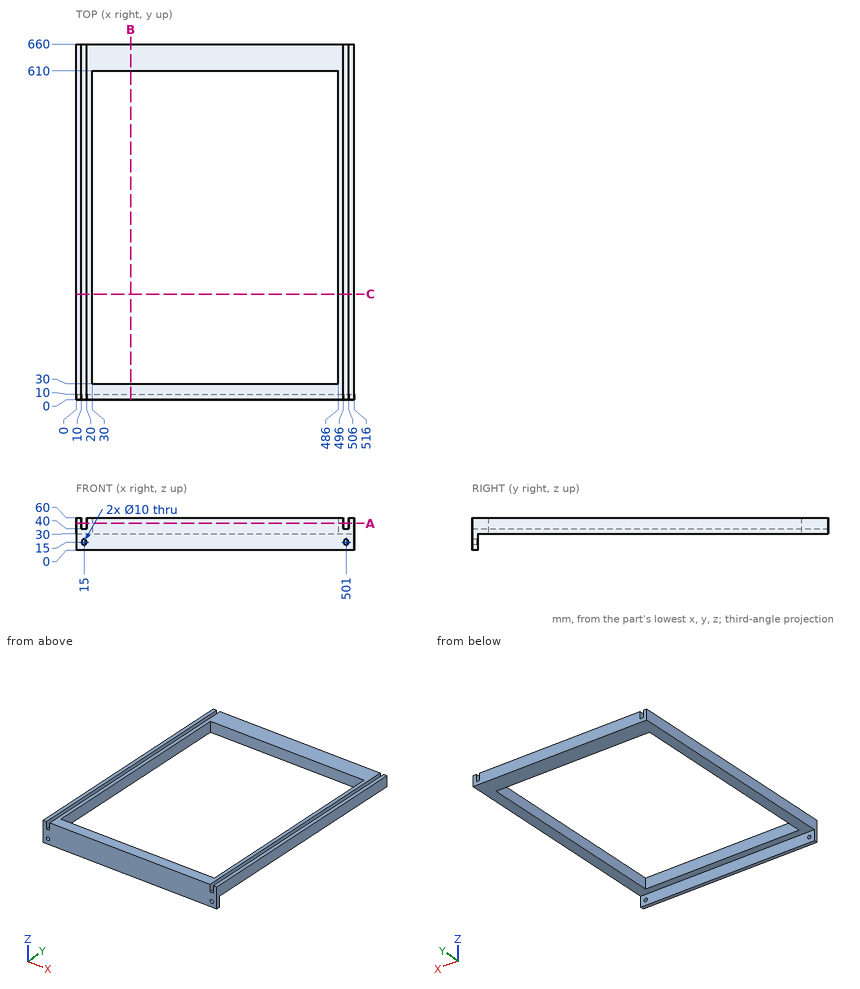
The figure shows three views and two pictorial views of one solid part (mm, origin at its lowest corner). Answer the questions. Coordinates: 2 decimals unless noted, no trailing zeros. Loops run counter-clockwise (first coordinate to the right, second up) from the corner with the lowest first, then second, coordinate; pieces in that order, holes last. Notation, with made-up numbers: (89, 59.5) - (100, 59.5) arc R12 ccw to (100, 82.5) - close; hole circle Ø4 at (12.25, 35.5). An arc over 180 degrees is marked (long way). Use a Markdown table: item, result. Add a question column.
1) The part is cut by section C-C, the plane y = 196. Give the vertices of the cut face in (x, z), and give its area (3 significant figures).
2) Given pin 1 (15 mm diameter, centred on x = 305, z = 18.5, fed in from +Y); pin 2 (5 mm diameter, centred on x = 13.5, y = 492.5, fed in from +Z), each flat-ended and moving along its own axis, determine where each tip first touches the part or whether it passes through.
3) The part is cut by section A-A, the plane z = 49.5. Give the vertices of the cut face in (x, y).
4) The part is cut by section B-B, the plane x = 101.5. Give the vertices of the cut face in (y, z), and give its area (3 significant figures).
5) Find the intervals of material crossed by line 1 (X direction, y = 317, z = 54); line 2 (Z direction, x = 15, y = 2); line 3 (Y direction, x = 103, z = 52), in increasing order.
Here are the results:
| question | item | result |
|---|---|---|
| 1 | outline | (0, 30) - (30, 30) - (30, 60) - (20, 60) - (20, 40) - (10, 40) - (10, 60) - (0, 60) - close; (486, 30) - (516, 30) - (516, 60) - (506, 60) - (506, 40) - (496, 40) - (496, 60) - (486, 60) - close |
| 1 | area | 1,400 mm^2 |
| 2 | pin 1 | stops at y = 10 |
| 2 | pin 2 | stops at z = 40 |
| 3 | outline | (0, 0) - (10, 0) - (10, 660) - (0, 660) - close; (20, 0) - (496, 0) - (496, 660) - (20, 660) - close; (506, 0) - (516, 0) - (516, 660) - (506, 660) - close; hole (30, 30) - (486, 30) - (486, 610) - (30, 610) - close |
| 4 | outline | (0, 0) - (10, 0) - (10, 30) - (30, 30) - (30, 60) - (0, 60) - close; (610, 30) - (660, 30) - (660, 60) - (610, 60) - close |
| 4 | area | 2,700 mm^2 |
| 5 | line 1 | x = 0 to 10, 20 to 30, 486 to 496, 506 to 516 |
| 5 | line 2 | z = 0 to 10, 20 to 40 |
| 5 | line 3 | y = 0 to 30, 610 to 660 |
